The model under review builds one solid part; all positions refer to its coordinate system, in mm. A direction names the side the tool comes from. Round coordinates to 2 decimals unless told otherwise and drop trailing zeros. Write each loop counter-clockwise with the first axis right and the second up, starting at its lowest first coordinate (ties: lowest second). Pieces come first, ordered by that corner, then holes. Notation, with made-up numbers: (59.5, -30) - (77.5, -30) arc R27 ccw to (77.5, -13) - close; hole circle Ø11 at (47, 61.5). An arc over 180 degrees is marked (long way). Return JSON: item names as keys, results as strings.
from build123d import *

# Parameters (mm, degrees)
ESQUISSE1_R             = 150
BOSS_EXTRU_1_DEPTH      = 12.7
ESQUISSE2_R             = 2
ENL_V_MAT_EXTRU_1_DEPTH = 12.7
ESQUISSE6_W             = 35
ESQUISSE6_H             = 29
ENL_V_MAT_EXTRU_2_DEPTH = 6.35


with BuildPart() as part:
    # Esquisse1 → Boss.-Extru.1 (new body)
    with BuildSketch(Plane.XY):
        Circle(ESQUISSE1_R)
    extrude(amount=BOSS_EXTRU_1_DEPTH)

    # Esquisse2 → Enlèv. mat.-Extru.1 (cut)
    with BuildSketch(Plane.XY.offset(12.7)):
        with Locations((-33, 48.25)):
            Circle(ESQUISSE2_R)
        with Locations((33, 48.25)):
            Circle(ESQUISSE2_R)
        with Locations((-33, -48.25)):
            Circle(ESQUISSE2_R)
        with Locations((33, -48.25)):
            Circle(ESQUISSE2_R)
    extrude(amount=-ENL_V_MAT_EXTRU_1_DEPTH, mode=Mode.SUBTRACT)

    # Esquisse6 → Enlèv. mat.-Extru.2 (cut)
    with BuildSketch(Plane.XY.offset(12.7)):
        with Locations((35.5, 110.228215567)):
            Rectangle(ESQUISSE6_W, ESQUISSE6_H)
        Polygon((73.90306654, -63.452565052), (56.40306654, -93.763454184), (81.51780325, -108.263454184), (99.01780325, -77.952565052), align=None)
        Polygon((-109.40306654, -1.964761383), (-91.90306654, -32.275650515), (-117.01780325, -46.775650515), (-134.51780325, -16.464761383), align=None)
    extrude(amount=-ENL_V_MAT_EXTRU_2_DEPTH, mode=Mode.SUBTRACT)


solid = part.part
(1) Clearance check with flat-ended pins moving along their axes: pin 1 Ø5 at (x, z) = (40.5, 9.5) entering from +Y; pin 2 Ø3.5 at (x, y) = (33, 48.25) entering from +Z; pin 3 Ø6 at (x, y) = (80.5, -10) entering from -Z; pin 4 Ø7 at (y, z) = (117, 9.5) entering from -X. State where each tip first meets the part, or that it passes through.
Filled in:
{"pin 1": "stops at y = 145.11", "pin 2": "passes through", "pin 3": "stops at z = 0", "pin 4": "stops at x = -98.07"}
(2) Mouldability with a two-part tool opening along X and no side actions: class faces 1 (the flat face through (-2, 2, 12.7)), 2 (the cylindrical face through (-19.527, 148.724, 6.261)), 3 (the flat face through (68.78, -100.91, 9.57)) as released by +X, released by -X, zero draft, split by the parting line, or undercut.
Filled in:
{"face 1": "zero draft", "face 2": "split by the parting line", "face 3": "undercut"}
(3) Add section A-A (z = 8.75). Write out the cut boundary in (x, y).
Filled in:
{"outline": "circle Ø300 at (0, 0); hole (-134.52, -16.46) - (-117.02, -46.78) - (-91.9, -32.28) - (-109.4, -1.96) - close; hole circle Ø4 at (-33, -48.25); hole circle Ø4 at (-33, 48.25); hole (18, 95.73) - (53, 95.73) - (53, 124.73) - (18, 124.73) - close; hole circle Ø4 at (33, -48.25); hole circle Ø4 at (33, 48.25); hole (56.4, -93.76) - (81.52, -108.26) - (99.02, -77.95) - (73.9, -63.45) - close"}
(4) Add section C-C (y = 100). Write out the cut boundary in (x, z).
Filled in:
{"outline": "(-111.8, 0) - (111.8, 0) - (111.8, 12.7) - (53, 12.7) - (53, 6.35) - (18, 6.35) - (18, 12.7) - (-111.8, 12.7) - close"}
(5) Wall thickness on line 1 (Y direction, x = 33, z = 7.75); line 2 (X direction, y = -50, z = 5.75); line 3 (Y direction, x = 33, z = 6): over which ranges is each line inside the solid? List them lowest first.
Filled in:
{"line 1": "y = -146.32 to -50.25, -46.25 to 46.25, 50.25 to 95.73, 124.73 to 146.32", "line 2": "x = -141.42 to -33.97, -32.03 to 32.03, 33.97 to 141.42", "line 3": "y = -146.32 to -50.25, -46.25 to 46.25, 50.25 to 146.32"}
(6) Add section B-B (x = 63). Write out the cut boundary in (y, z).
Filled in:
{"outline": "(-136.13, 0) - (136.13, 0) - (136.13, 12.7) - (-82.34, 12.7) - (-82.34, 6.35) - (-97.57, 6.35) - (-97.57, 12.7) - (-136.13, 12.7) - close"}
(7) For faces 4 (the flat face through (-100.776, -16.908, 9.569)), 5 (the flat face through (-2, 2, 0)), list the 3-axis set-ups (+Z, -Z, +X, -X, +Y, -Y) from which the entire face can be reached by the end or side of a thin tool; tool diameter is ignored.
Filled in:
{"face 4": "+Z", "face 5": "-Z, +X, -X, +Y, -Y"}
(8) Add section D-D (y = 42.5). Write out the cut boundary in (x, z), plus the area to 3 significant figures.
Filled in:
{"outline": "(-143.85, 0) - (143.85, 0) - (143.85, 12.7) - (-143.85, 12.7) - close", "area": "3,650 mm2"}
